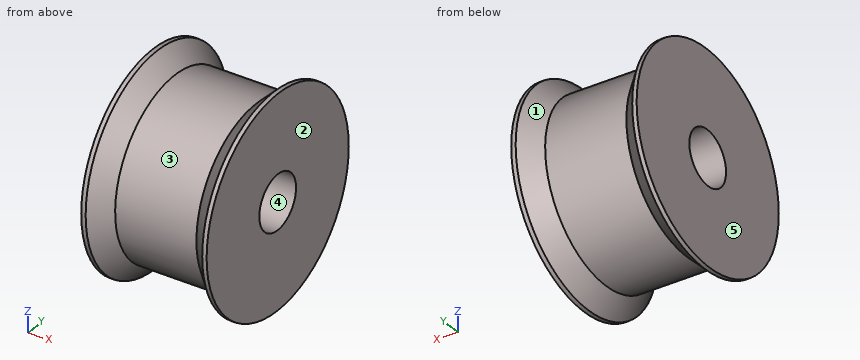
```python
from build123d import *

# Parameters (mm, degrees)
SKETCH3_R          = 3.1
CUT_EXTRUDE1_DEPTH = 14.2


with BuildPart() as part:
    # Sketch2 → Revolve1 (revolve)
    with BuildSketch(Plane(origin=(0, 0, 0), x_dir=(1, 0, 0), z_dir=(0, 1, 0))):
        Polygon((-7.1, 12), (-6.6, 12), (-4.6, 10), (4.6, 10), (6.6, 12), (7.1, 12), (7.1, 0), (-7.1, 0), align=None)
    revolve(axis=Axis((7.1, 0, 0), (-1, 0, 0)))

    # Sketch3 → Cut-Extrude1 (cut)
    with BuildSketch(Plane.ZY.offset(7.1)):
        Circle(SKETCH3_R)
    extrude(amount=-CUT_EXTRUDE1_DEPTH, mode=Mode.SUBTRACT)


solid = part.part
```
Geometry check sheet. Reference: the model listing, model coordinates, mm. Face numbers are marked on the shaded views. A direction names the side the tool comes from. Give positions to 0.01 mm unless a question says otherwise; leave off trailing zeros. Order: outer loops, then holes, each group sorted by start corner. A loop starts at its lowest first (then second) coordinate and runs counter-clockwise, first axis right, second up. Notation, with made-up numbers: (48.25, 18.5) - (66.25, 18.5) arc R17 ccw to (66.25, 32.5) - close; hole circle Ø8 at (65.25, -36). An arc over 180 degrees is marked (long way). Answer in a Markdown table with one row per item. Add a question column.
Q1. Cross-section at D-D, the plane x = -6. Enter the section's corners in (y, z).
Q2. Material ranges on probe 1 along Y at (x, z) = (1, 0); probe 2 along Y at (x, z) = (-3, 1); probe 3 along X at (y, z) = (-0.5, 10.5), recorded low to high. Write a range as from..to.
Q3. Mould release check, pull along Z, two halves, no side actions. Record for the marked faces 3, 4 and 5: pulls with the +Z half, pulls with the -Z half, needs draft (parallel to the pull), parting line crosses it, or undercut.
Q4. Gauge pin test, flat ends, axial feed: pin 1 (5 mm diameter, centred on x = 5, z = -9, fed in from +Y); pin 2 (1 mm diameter, centred on x = 3.5, z = 1.5, fed in from -Y); pin 3 (1.5 mm diameter, centred on x = -1, y = 2, fed in from +Z). Record the tip position at first contact, or that the pin passes through.
Q5. Cross-section at C-C, the plane x = 6.25. Enter the section's corners in (y, z), then the cut area to 3 significant figures.
Q6. Tool access check on the marked faces 1 and 2. Record the directions out of +Z, -Z, +X, -X, +Y, -Y that give a thin tool (end or side, any length) a straight path to the whole face; none if there is none.
Q7. Cross-section at A-A, the plane z = 0. Enter the section's corners in (x, y), then the cut area to 3 significant figures.
Check values:
| question | item | result |
|---|---|---|
| 1 | outline | circle Ø22.8 at (0, 0); hole circle Ø6.2 at (0, 0) |
| 2 | probe 1 | y = -10..-3.1, 3.1..10 |
| 2 | probe 2 | y = -9.95..-2.93, 2.93..9.95 |
| 2 | probe 3 | x = -7.1..-5.11, 5.11..7.1 |
| 3 | face 3 | parting line crosses it |
| 3 | face 4 | undercut |
| 3 | face 5 | needs draft |
| 4 | pin 1 | stops at y = 9.69 |
| 4 | pin 2 | stops at y = -9.95 |
| 4 | pin 3 | stops at z = 9.92 |
| 5 | outline | circle Ø23.3 at (0, 0); hole circle Ø6.2 at (0, 0) |
| 5 | area | 396 mm^2 |
| 6 | face 1 | none |
| 6 | face 2 | +Z, -Z, +X, +Y, -Y |
| 7 | outline | (-7.1, -12) - (-6.6, -12) - (-4.6, -10) - (4.6, -10) - (6.6, -12) - (7.1, -12) - (7.1, -3.1) - (-7.1, -3.1) - close; (-7.1, 3.1) - (7.1, 3.1) - (7.1, 12) - (6.6, 12) - (4.6, 10) - (-4.6, 10) - (-6.6, 12) - (-7.1, 12) - close |
| 7 | area | 208 mm^2 |
